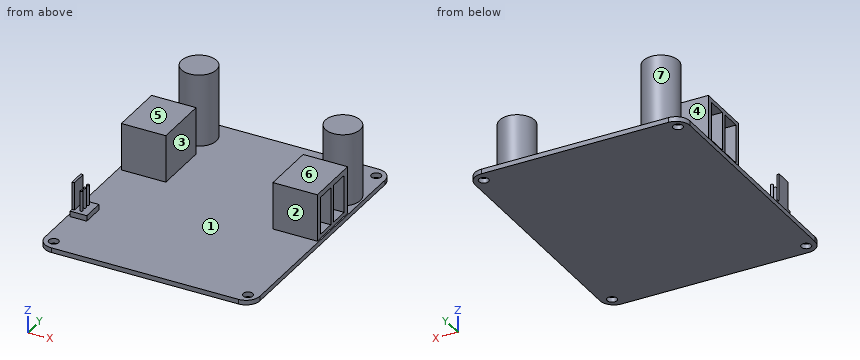
```python
from build123d import *

# Parameters (mm, degrees)
SKETCH1_R           = 1.75
BOSS_EXTRUDE1_DEPTH = 1.7
SKETCH2_R           = 6.3
BOSS_EXTRUDE2_DEPTH = 26
SKETCH3_W           = 16
SKETCH3_H           = 20
BOSS_EXTRUDE3_DEPTH = 17
SKETCH4_W           = 13.854016079
SKETCH4_H           = 7.22206482
SKETCH4_H_2         = 7.167084928
CUT_EXTRUDE1_DEPTH  = 13
SKETCH5_W           = 13.539526547
SKETCH5_H           = 7.062187725
SKETCH5_H_2         = 6.849826242
CUT_EXTRUDE2_DEPTH  = 13
SKETCH6_W           = 6
SKETCH6_H           = 8
BOSS_EXTRUDE5_DEPTH = 12
SKETCH7_R           = 0.5
CUT_EXTRUDE3_DEPTH  = 10
SKETCH8_W           = 2.826271855
SKETCH8_H           = 5.802654235
CUT_EXTRUDE4_DEPTH  = 123.76480237


with BuildPart() as part:
    # Sketch1 → Boss-Extrude1 (new body)
    with BuildSketch(Plane.XY):
        with BuildLine():
            Line((5, 0), (72.37, 0))
            ThreePointArc((72.37, 0), (75.905533906, 1.464466094), (77.37, 5))
            Line((77.37, 5), (77.37, 87.67))
            ThreePointArc((77.37, 87.67), (75.905533906, 91.205533906), (72.37, 92.67))
            Line((72.37, 92.67), (5, 92.67))
            ThreePointArc((5, 92.67), (1.464466094, 91.205533906), (0, 87.67))
            Line((0, 87.67), (0, 5))
            ThreePointArc((0, 5), (1.464466094, 1.464466094), (5, 0))
        make_face()
        with Locations((73.62, 88.72)):
            Circle(SKETCH1_R, mode=Mode.SUBTRACT)
        with Locations(Location((3.75, 88.72, 0), (0, 0, 180))):
            Circle(SKETCH1_R, mode=Mode.SUBTRACT)
        with Locations((3.75, 3.95)):
            Circle(SKETCH1_R, mode=Mode.SUBTRACT)
        with Locations(Location((73.62, 3.95, 0), (0, 0, 180))):
            Circle(SKETCH1_R, mode=Mode.SUBTRACT)
    extrude(amount=BOSS_EXTRUDE1_DEPTH)

    # Sketch2 → Boss-Extrude2 (add)
    with BuildSketch(Plane.XY.offset(1.7)):
        with Locations(Location((12.6, 83.67, 0), (0, 0, 180))):
            Circle(SKETCH2_R)
        with Locations(Location((70.37, 72.67, 0), (0, 0, 180))):
            Circle(SKETCH2_R)
    extrude(amount=BOSS_EXTRUDE2_DEPTH)

    # Sketch3 → Boss-Extrude3 (add)
    with BuildSketch(Plane.XY.offset(1.7)):
        with Locations((68.875904293, 53.835144036)):
            Rectangle(SKETCH3_W, SKETCH3_H)
        with Locations((9.163906292, 63.368262293)):
            Rectangle(SKETCH3_W, SKETCH3_H)
    extrude(amount=BOSS_EXTRUDE3_DEPTH)

    # Sketch4 → Cut-Extrude1 (cut)
    with BuildSketch(Plane.ZY.offset(-1.163906292)):
        with Locations((10.29633171, 67.739791882)):
            Rectangle(SKETCH4_W, SKETCH4_H)
        with Locations((10.29633171, 58.701978818)):
            Rectangle(SKETCH4_W, SKETCH4_H_2)
    extrude(amount=-CUT_EXTRUDE1_DEPTH, mode=Mode.SUBTRACT)

    # Sketch5 → Cut-Extrude2 (cut)
    with BuildSketch(Plane(origin=(76.875904293, 0, 0), x_dir=(0, 0, -1), z_dir=(1, 0, 0))):
        with Locations((-9.923616317, 58.019849725)):
            Rectangle(SKETCH5_W, SKETCH5_H)
        with Locations((-9.923616317, 49.287198962)):
            Rectangle(SKETCH5_W, SKETCH5_H_2)
    extrude(amount=-CUT_EXTRUDE2_DEPTH, mode=Mode.SUBTRACT)

    # Sketch6 → Boss-Extrude5 (add)
    with BuildSketch(Plane.XY.offset(1.7)):
        with Locations((3.883233482, 24)):
            Rectangle(SKETCH6_W, SKETCH6_H)
    extrude(amount=BOSS_EXTRUDE5_DEPTH)

    # Sketch7 → Cut-Extrude3 (cut)
    with BuildSketch(Plane.XY.offset(13.7)):
        Polygon((6.883233482, 28), (0.883233482, 28), (0.883233482, 27.053748642), (1.764591458, 27.053748642), (1.764591458, 21.251094407), (0.883233482, 21.251094407), (0.883233482, 20), (6.883233482, 20), align=None)
        with Locations((3.883233482, 22.03910918)):
            Circle(SKETCH7_R, mode=Mode.SUBTRACT)
        with Locations((3.883233482, 24.152421525)):
            Circle(SKETCH7_R, mode=Mode.SUBTRACT)
        with Locations((3.883233482, 26.265733869)):
            Circle(SKETCH7_R, mode=Mode.SUBTRACT)
    extrude(amount=-CUT_EXTRUDE3_DEPTH, mode=Mode.SUBTRACT)

    # Sketch8 → Cut-Extrude4 (cut, through all)
    with BuildSketch(Plane(origin=(1.764591458, 0, 0), x_dir=(0, 0, -1), z_dir=(1, 0, 0))):
        with Locations((-12.286864073, 24.152421524)):
            Rectangle(SKETCH8_W, SKETCH8_H)
    extrude(amount=CUT_EXTRUDE4_DEPTH, mode=Mode.SUBTRACT)


solid = part.part
```
Could you check a few things on this model? Use its own coordinates, in mm. Face numbers are marked on the shaded views. A direction names the side the tool comes from. Give positions to 0.01 mm unless a question says otherwise; leave off trailing zeros. Loops run counter-clockwise (first coordinate to the right, second up) from the corner with the lowest first, then second, coordinate; pieces in that order, holes last. Notation, with made-up numbers: (64.25, -0.5) - (122.25, -0.5) arc R23 cw to (122.25, 27.5) - close; hole circle Ø8 at (42, 56). An arc over 180 degrees is marked (long way). Use one line per item in the form item = value.
1. I want a section at C-C (y = 88.72). Please give me the cut outline in (x, z), and give its area (3 significant figures).
Response values:
outline = (0.11, 0) - (2, 0) - (2, 1.7) - (0.11, 1.7) - close; (5.5, 0) - (71.87, 0) - (71.87, 1.7) - (16.37, 1.7) - (16.37, 27.7) - (8.83, 27.7) - (8.83, 1.7) - (5.5, 1.7) - close; (75.37, 0) - (77.26, 0) - (77.26, 1.7) - (75.37, 1.7) - close
area = 315 mm²
2. I want a section at D-D (z = 22.75). Please give me the cut outline in (x, y), and give its area (3 significant figures).
Response values:
outline = circle Ø12.6 at (12.6, 83.67); circle Ø12.6 at (70.37, 72.67)
area = 249 mm²
3. I need wall thicknesses on probe 1 along Y at (x, z) = (3.75, 1.2); probe 2 along X at (y, z) = (88.72, 1.1); probe 3 along Z at (x, y) = (72, 29). Which ranges of each line are inside material? Lowest first, please.
Response values:
probe_1 = 0.16 to 2.2, 5.7 to 86.97, 90.47 to 92.51
probe_2 = 0.11 to 2, 5.5 to 71.87, 75.37 to 77.26
probe_3 = 0 to 1.7
4. I want a section at B-B (x = 12.6). Please give me the cut outline in (y, z).
Response values:
outline = (0, 0) - (92.67, 0) - (92.67, 1.7) - (89.97, 1.7) - (89.97, 27.7) - (77.37, 27.7) - (77.37, 1.7) - (73.37, 1.7) - (73.37, 18.7) - (53.37, 18.7) - (53.37, 1.7) - (0, 1.7) - close; hole (55.12, 3.37) - (62.29, 3.37) - (62.29, 17.22) - (55.12, 17.22) - close; hole (64.13, 3.37) - (71.35, 3.37) - (71.35, 17.22) - (64.13, 17.22) - close
5. I want a section at A-A (x = 73.62). Please give me the cut outline in (y, z), and give its area (3 significant figures).
Response values:
outline = (0.16, 0) - (2.2, 0) - (2.2, 1.7) - (0.16, 1.7) - close; (5.7, 0) - (86.97, 0) - (86.97, 1.7) - (78.07, 1.7) - (78.07, 27.7) - (67.27, 27.7) - (67.27, 1.7) - (63.84, 1.7) - (63.84, 18.7) - (43.84, 18.7) - (43.84, 1.7) - (5.7, 1.7) - close; (90.47, 0) - (92.51, 0) - (92.51, 1.7) - (90.47, 1.7) - close; hole (45.86, 3.15) - (52.71, 3.15) - (52.71, 16.69) - (45.86, 16.69) - close; hole (54.49, 3.15) - (61.55, 3.15) - (61.55, 16.69) - (54.49, 16.69) - close
area = 577 mm²
6. Thinking about a two-plate mould opening in X: for the marked faces 1 and 2, which applies, released by +X, released by -X, zero draft, split by the parting line, or undercut?
Response values:
face_1 = undercut
face_2 = zero draft
7. On a 3-axis mill with a long thin cutter (end or side, diameter ignored), from which of +Z, -Z, +X, -X, +Y, -Y can I reach the whole of each face in a straight line? I mean the marked faces 3, 4, 5, 6 and 7. Say none if no direction works.
Response values:
face_3 = +Z, -Y
face_4 = +Z, -X
face_5 = +Z, -X, -Y
face_6 = +Z, +X, -X, -Y
face_7 = +Z
8. I'm going to push flat-ended pins straight in: pin 1 Ø4 at (x, y) = (73.62, 3.95) entering from +Z; pin 2 Ø5 at (y, z) = (63, 5) entering from +X; pin 3 Ø2 at (x, z) = (11.5, 20) entering from +Y. Where does each tip first touch, or does it pass through?
Response values:
pin_1 = 1.7
pin_2 = 76.88
pin_3 = 89.97
